Geometry check sheet. Reference: drawing and pictorial views, mm from the part's lowest x, y, z. Give positions to 0.01 mm unless a question says otherwise; leave off trailing zeros. Write each loop counter-clockwise with the first axis right and the second up, starting at its lowest first coordinate (ties: lowest second). Pieces come first, ordered by that corner, then holes. Notation, with made-up numbers: (78.5, 4.5) - (99.5, 4.5) arc R36 ccw to (99.5, 43.5) - close; hole circle Ø2 at (26, 61.5). An arc over 180 degrees is marked (long way). Write item = value, one per line. Start each with the question number.
(1) Thickness scan on L1, parallel to Y at x = 7.5, z = 7; L2, parallel to X at y = 8, z = 58; L3, parallel to Z at x = 8.25, y = 6.5. Record the ranges inside material, lowest first.
(2) Section check C-C, the plane z = 48. Enter the section's corners in (x, y), plus the area to 3 significant figures.
(3) Section check D-D, the plane y = 4.5. Enter the section's corners in (x, z), plus the area to 3 significant figures.
(4) Section check A-A, the plane y = 7.5. Enter the section's corners in (x, z).
(5) Depth check by flat-ended pin: pin 1 Ø3 at (x, y) = (7.5, 7.5) entering from +Z; pin 2 Ø4.5 at (x, y) = (7.5, 7.5) entering from +Z; pin 3 Ø5 at (x, z) = (11, 8.5) entering from -Y; pin 4 Ø6 at (y, z) = (11.5, 53) entering from -X. Enter the tip coordinate at first touch or a pass-through.
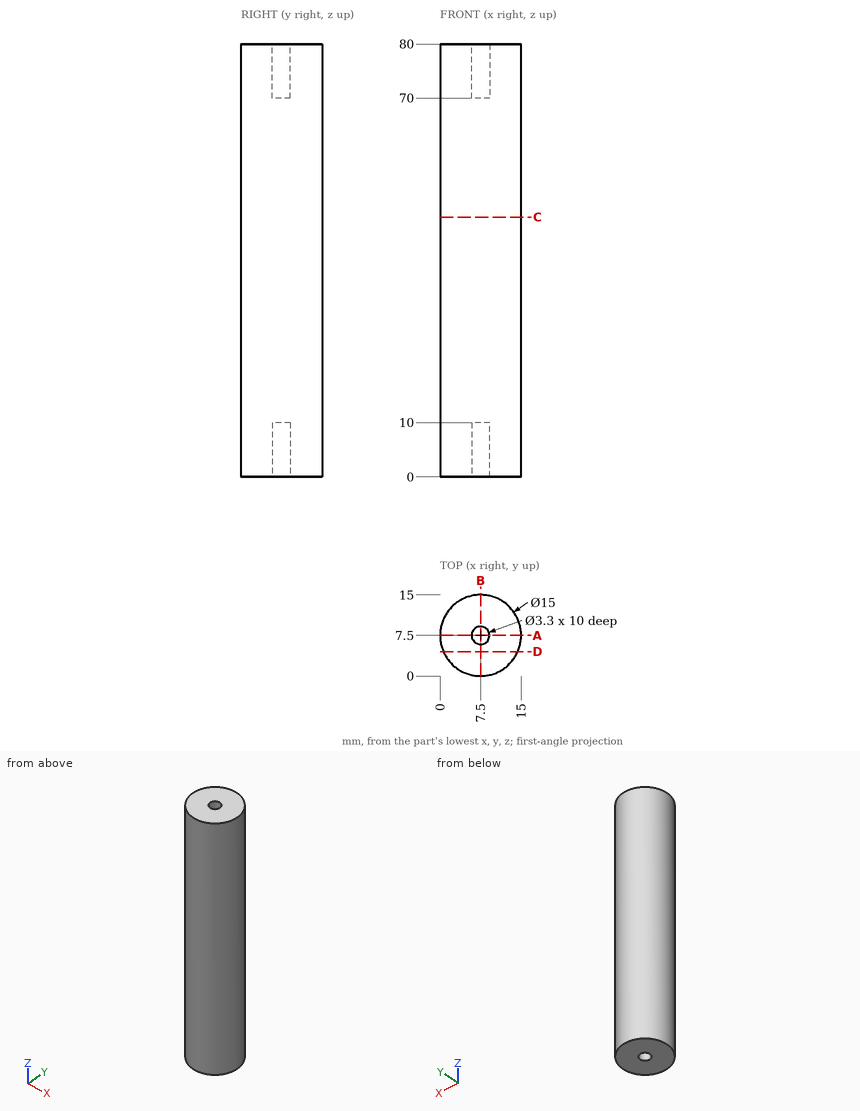
Model answer:
q1.L1 = 0 to 5.85, 9.15 to 15
q1.L2 = 0.02 to 14.98
q1.L3 = 10 to 70
q2.outline = circle Ø15 at (7.5, 7.5)
q2.area = 177 mm²
q3.outline = (0.63, 0) - (14.37, 0) - (14.37, 80) - (0.63, 80) - close
q3.area = 1,100 mm²
q4.outline = (0, 0) - (5.85, 0) - (5.85, 10) - (9.15, 10) - (9.15, 0) - (15, 0) - (15, 80) - (9.15, 80) - (9.15, 70) - (5.85, 70) - (5.85, 80) - (0, 80) - close
q5.pin_1 = 70
q5.pin_2 = 80
q5.pin_3 = 0.07
q5.pin_4 = 0.07
